```python
from build123d import *

# Parameters (mm, degrees)
BOSS_EXTRUDE1_DEPTH  = 6.35
SKETCH1_W            = 69.85
SKETCH1_H            = 67.056
BOSS_EXTRUDE2_DEPTH  = 31.75
SKETCH3_R            = 103.505
SKETCH3_R_2          = 90.805
BOSS_EXTRUDE3_DEPTH  = 38.1
BOSS_EXTRUDE4_START  = -3.175
SKETCH3_2_R          = 103.505
BOSS_EXTRUDE4_DEPTH  = 3.175
BOSS_EXTRUDE5_REACH  = 154.086
SKETCH1_3_W          = 69.85
SKETCH1_3_H          = 67.056
BOSS_EXTRUDE6_DEPTH  = 31.75
BOSS_EXTRUDE7_DEPTH  = 21.59
SKETCH8_R            = 4.445
BOSS_EXTRUDE8_DEPTH  = 3.81
FILLET1_R            = 3.81
FILLET1_OF_MIRROR3_R = 3.81
SKETCH9_W            = 40.64
SKETCH9_H            = 40.64
BOSS_EXTRUDE9_DEPTH  = 50.8
SKETCH10_R           = 19.05
BOSS_EXTRUDE10_DEPTH = 68.58


with BuildPart() as part:
    # Sketch2 → Boss-Extrude1 (new body)
    with BuildSketch(Plane.XY):
        with BuildLine():
            Line((-90.805, 0), (-34.925, 0))
            Line((-34.925, 0), (-34.925, -33.528))
            Line((-34.925, -33.528), (34.925, -33.528))
            Line((34.925, -33.528), (34.925, 0))
            Line((34.925, 0), (90.805, 0))
            ThreePointArc((90.805, 0), (0, -90.805), (-90.805, 0))
        make_face()
    extrude(amount=BOSS_EXTRUDE1_DEPTH)

    # Sketch1 → Boss-Extrude2 (add)
    with BuildSketch(Plane.XY):
        Rectangle(SKETCH1_W, SKETCH1_H)
    extrude(amount=BOSS_EXTRUDE2_DEPTH)

    # Sketch3 → Boss-Extrude3 (add)
    with BuildSketch(Plane.XY.offset(-31.75)):
        with Locations(Location((0, 0, 0), (0, 0, 180))):
            Circle(SKETCH3_R)
        Circle(SKETCH3_R_2, mode=Mode.SUBTRACT)
    extrude(amount=BOSS_EXTRUDE3_DEPTH)

    # Sketch3<2> → Boss-Extrude4 (add)
    with BuildSketch(Plane.XY.offset(-31.75).offset(BOSS_EXTRUDE4_START)):
        with Locations(Location((0, 0, 0), (0, 0, 180))):
            Circle(SKETCH3_2_R)
    extrude(amount=BOSS_EXTRUDE4_DEPTH)

    # Boss-Extrude5: up to this face of the body (flat: up to its plane)
    boss_extrude5_end = Plane(part.part.faces().sort_by_distance((0, 0, -31.75))[0])
    # Sketch5 → Boss-Extrude5 (add, up to the picked face)
    with BuildSketch(Plane.XY.offset(6.35), mode=Mode.PRIVATE) as boss_extrude5_sk1:
        with BuildLine():
            Line((-90.805, 0), (-34.925, 0))
            Line((-34.925, 0), (-34.925, -6.35))
            Line((-34.925, -6.35), (-90.582699921, -6.35))
            ThreePointArc((-90.582699921, -6.35), (-90.749407963, -3.176944968), (-90.805, 0))
        make_face()
    boss_extrude5_tool1 = split(extrude(boss_extrude5_sk1.sketch, amount=-BOSS_EXTRUDE5_REACH, mode=Mode.PRIVATE), bisect_by=boss_extrude5_end, keep=Keep.BOTH, mode=Mode.PRIVATE)
    # Sketch5 → Boss-Extrude5 (add, up to the picked face)
    with BuildSketch(Plane.XY.offset(6.35), mode=Mode.PRIVATE) as boss_extrude5_sk2:
        with BuildLine():
            Line((34.925, 0), (90.805, 0))
            ThreePointArc((90.805, 0), (90.749407963, -3.176944968), (90.582699921, -6.35))
            Line((90.582699921, -6.35), (34.925, -6.35))
            Line((34.925, -6.35), (34.925, 0))
        make_face()
    boss_extrude5_tool2 = split(extrude(boss_extrude5_sk2.sketch, amount=-BOSS_EXTRUDE5_REACH, mode=Mode.PRIVATE), bisect_by=boss_extrude5_end, keep=Keep.BOTH, mode=Mode.PRIVATE)
    # Sketch5 → Boss-Extrude5 (add, up to the picked face)
    with BuildSketch(Plane.XY.offset(6.35), mode=Mode.PRIVATE) as boss_extrude5_sk3:
        Polygon((0, 33.528), (3.175, 33.528), (3.175, 94.488), (-3.175, 94.488), (-3.175, 33.528), align=None)
    boss_extrude5_tool3 = split(extrude(boss_extrude5_sk3.sketch, amount=-BOSS_EXTRUDE5_REACH, mode=Mode.PRIVATE), bisect_by=boss_extrude5_end, keep=Keep.BOTH, mode=Mode.PRIVATE)
    add(boss_extrude5_tool1.solids().sort_by(Axis((-62.828007, -3.172893, 6.35), (0, 0, -1)))[0])
    add(boss_extrude5_tool2.solids().sort_by(Axis((62.828007, -3.172893, 6.35), (0, 0, -1)))[0])
    add(boss_extrude5_tool3.solids().sort_by(Axis((0, 64.008, 6.35), (0, 0, -1)))[0])

    # Sketch1<3> → Boss-Extrude6 (add)
    with BuildSketch(Plane.XY):
        Rectangle(SKETCH1_3_W, SKETCH1_3_H)
    extrude(amount=-BOSS_EXTRUDE6_DEPTH)

    # Sketch6 → Revolve1 (revolve)
    with BuildSketch(Plane(origin=(0, 0, 0), x_dir=(1, 0, 0), z_dir=(0, 1, 0))):
        Polygon((-103.505, -6.35), (-99.695, -25.4), (-95.885, -6.35), align=None)
    revolve(axis=Axis((0, 0, 0), (0, 0, 1)))

    # Sketch7 → Boss-Extrude7 (add)
    with BuildSketch(Plane.XY.offset(6.35)):
        with BuildLine():
            ThreePointArc((-13.17823844, -98.820175352), (-13.067443237, -38.631075363), (-49.51802331, -86.527789712))
            ThreePointArc((-49.51802331, -86.527789712), (-45.608408723, -88.650809803), (-41.607971429, -90.597294323))
            ThreePointArc((-41.607971429, -90.597294323), (-14.084798914, -41.638667826), (-21.934434586, -97.252113624))
            ThreePointArc((-21.934434586, -97.252113624), (-17.573834418, -98.133854346), (-13.17823844, -98.820175352))
        make_face()
    extrude(amount=BOSS_EXTRUDE7_DEPTH)

    # Sketch8 → Boss-Extrude8 (add)
    with BuildSketch(Plane(origin=(34.925, 0, 0), x_dir=(0, 0, -1), z_dir=(1, 0, 0))):
        with Locations(Location((-16.51, 12.7, 0), (0, 0, 180))):
            Circle(SKETCH8_R)
        with Locations(Location((-16.51, -12.7, 0), (0, 0, 180))):
            Circle(SKETCH8_R)
    boss_extrude8 = extrude(amount=BOSS_EXTRUDE8_DEPTH)

    # Fillet1
    fillet1_edges = [part.edges().sort_by_distance(p)[0] for p in [
        (38.735, 12.7, 12.065),
        (38.735, -12.7, 12.065),
    ]]
    fillet(fillet1_edges, radius=FILLET1_R - 0.0001)  # a hair under: the kernel refuses the full size

    # Mirror3: Boss-Extrude8 across plane
    add(boss_extrude8.mirror(Plane(origin=(0, 0, 0), x_dir=(0, 0, 1), z_dir=(1, 0, 0))))

    # Fillet1 of Mirror3
    fillet1_of_mirror3_edges = [part.edges().sort_by_distance(p)[0] for p in [
        (-38.735, 12.7, 12.065),
        (-38.735, -12.7, 12.065),
    ]]
    fillet(fillet1_of_mirror3_edges, radius=FILLET1_OF_MIRROR3_R - 0.0001)  # a hair under: the kernel refuses the full size

    # Sketch9 → Boss-Extrude9 (add)
    with BuildSketch(Plane.XY.offset(31.75)):
        Rectangle(SKETCH9_W, SKETCH9_H)
    extrude(amount=BOSS_EXTRUDE9_DEPTH)

    # Sketch10 → Boss-Extrude10 (add)
    with BuildSketch(Plane.XY.offset(82.55)):
        Circle(SKETCH10_R)
    extrude(amount=BOSS_EXTRUDE10_DEPTH)


solid = part.part
```
The listing builds one solid part. Answer for the finished solid, in the listing's coordinates (mm). A direction names the side the tool comes from. Round coordinates to 2 decimals unless told otherwise and drop trailing zeros. Loops run counter-clockwise (first coordinate to the right, second up) from the corner with the lowest first, then second, coordinate; pieces in that order, holes last. Notation, with made-up numbers: (11.5, -11) - (65.5, -11) arc R37 ccw to (65.5, 27) - close; hole circle Ø2 at (38, 15.5). An arc over 180 degrees is marked (long way). Use one line per item in the form item = value. Start each with the question number.
1. A tool of negligible diameter and unlimited length cuts with its end or side. For faces 1 (the face through (1, -49, -31.75)), 2 (the face through (-19, -40, 27.94)), 3 (the face through (0, 33.528, 8)), from which of +Z, -Z, +X, -X, +Y, -Y can it reach the whole face along a straight path? Write none if from no direction.
2. The part is cut by section C-C on z = 66. Determine the outline of the cut face in (x, y), then the cut area to 3 significant figures.
3. Consider line 1 (Z direction, x = 14, y = -45) (3 decimals); line 2 (Y direction, x = -14.5, z = 13); line 3 (Y direction, x = 84, z = -6). Determine where each line is inside the solid, lowest interval first. Write a range as [from, to].
4. Given pin 1 Ø16.5 at (x, y) = (-20, -70.5) entering from +Z; pin 2 Ø16 at (x, z) = (12.5, -9.5) entering from -Y; pin 3 Ø12 at (y, z) = (46, -13.5) entering from +X, each flat-ended and moving along its own axis, determine where each tip first touches the part or whether it passes through.
5. The part is cut by section A-A on z = -8.5. Determine the outline of the cut face in (x, y) (3 decimals), then the cut area to 3 significant figures.
6. For a pull along Y with two mould halves and no side action, classify faces 4 (the face through (13.474, -102.624, -14.576)), 5 (the face through (-46, 45, -31.75)), 6 (the face through (0, 0, 151.13)) as pulls with the +Y half, pulls with the -Y half, needs draft (parallel to the pull), parting line crosses it, or undercut.
Geometry check:
q1.face_1 = none
q1.face_2 = +Z, +X, -X, -Y
q1.face_3 = +Z
q2.outline = (-20.32, -20.32) - (20.32, -20.32) - (20.32, 20.32) - (-20.32, 20.32) - close
q2.area = 1,650 mm^2
q3.line_1 = [-34.925, -31.75], [0, 6.35]
q3.line_2 = [-101.14, -95.91], [-41.5, -38.18], [-33.53, 33.53], [96.13, 101.14]
q3.line_3 = [-60.48, -34.49], [-6.35, 0], [34.49, 60.48]
q4.pin_1 = 6.35
q4.pin_2 = -103.41
q4.pin_3 = 95.46
q5.outline = circle Ø207.01 at (0, 0); hole (-90.805, 0) - (-34.925, 0) - (-34.925, 33.528) - (-3.175, 33.528) - (-3.175, 90.749) arc R90.805 ccw to start; hole (-90.583, -6.35) arc R90.805 ccw to (90.583, -6.35) - (34.925, -6.35) - (34.925, -33.528) - (-34.925, -33.528) - (-34.925, -6.35) - close; hole (3.175, 33.528) - (34.925, 33.528) - (34.925, 0) - (90.805, 0) arc R90.805 ccw to (3.175, 90.749) - close
q5.area = 13,500 mm^2
q6.face_4 = parting line crosses it
q6.face_5 = undercut
q6.face_6 = needs draft
